```python
from build123d import *

# Parameters (mm, degrees)
SKETCH_1_R          = 2
EXTRUDE_1_DEPTH     = 8
EXTRUDE_2_DEPTH     = 39
EXTRUDE_3_DEPTH     = 35
SKETCH_4_R          = 4.5
CUT_EXTRUDE_1_DEPTH = 55
FILLET_1_R          = 1
CHAMFER_1_SIZE      = 0.2


with BuildPart() as part:
    # 草图1 → 凸台-拉伸1 (new body)
    with BuildSketch(Plane(origin=(0, 0, 0), x_dir=(0, 0, -1), z_dir=(1, 0, 0))):
        with BuildLine():
            Line((0, 4.5), (4.5, 4.5))
            Line((4.5, 4.5), (4.5, -4.5))
            Line((4.5, -4.5), (-1.5, -4.5))
            ThreePointArc((-1.5, -4.5), (-3.621320344, -3.621320344), (-4.5, -1.5))
            Line((-4.5, -1.5), (-4.5, 1.5))
            ThreePointArc((-4.5, 1.5), (-3.621320344, 3.621320344), (-1.5, 4.5))
            Line((-1.5, 4.5), (0, 4.5))
        make_face()
        Circle(SKETCH_1_R, mode=Mode.SUBTRACT)
    extrude(amount=EXTRUDE_1_DEPTH)

    # 草图2 → 凸台-拉伸2 (add)
    with BuildSketch(Plane(origin=(0, 0, -4.5), x_dir=(-1, 0, 0), z_dir=(0, 0, -1))):
        Polygon((-4, 10), (3.5, 10), (3.5, -10), (-11.5, -10), (-11.5, 10), align=None)
    extrude(amount=EXTRUDE_2_DEPTH)

    # 草图3 → 凸台-拉伸3 (add)
    with BuildSketch(Plane(origin=(0, 0, -43.5), x_dir=(-1, 0, 0), z_dir=(0, 0, -1))):
        with BuildLine():
            Line((2.5, 6.224949799), (2.5, -6.224949799))
            ThreePointArc((2.5, -6.224949799), (-4, -9), (-10.5, -6.224949799))
            Line((-10.5, -6.224949799), (-10.5, 6.224949799))
            ThreePointArc((-10.5, 6.224949799), (-4, 9), (2.5, 6.224949799))
        make_face()
    extrude(amount=EXTRUDE_3_DEPTH)

    # 草图4 → 切除-拉伸1 (cut)
    with BuildSketch(Plane(origin=(0, 0, -78.5), x_dir=(-1, 0, 0), z_dir=(0, 0, -1))):
        with Locations(Location((-4, 0, 0), (0, 0, 90))):
            Circle(SKETCH_4_R)
    extrude(amount=-CUT_EXTRUDE_1_DEPTH, mode=Mode.SUBTRACT)

    # 圆角1
    fillet_1_edges = [part.edges().sort_by_distance(p)[0] for p in [
        (4, -10, -4.5),
        (4, 10, -4.5),
        (4, 10, -43.5),
        (4, -10, -43.5),
    ]]
    fillet(fillet_1_edges, radius=FILLET_1_R - 0.0001)  # a hair under: the kernel refuses the full size

    # 倒角1
    chamfer_1_edges = [part.edges().sort_by_distance(p)[0] for p in [
        (-3.5, -10, -24),
        (11.5, -10, -24),
        (-3.5, 0, -4.5),
        (-3.5, 10, -24),
        (-3.5, 0, -43.5),
        (-3.5, 9.707136071, -4.792863929),
        (-3.5, 9.707136071, -43.207136071),
        (-3.5, -9.707136071, -43.207136071),
        (-3.5, -9.707136071, -4.792863929),
        (11.5, 0, -4.5),
        (11.5, 0, -43.5),
        (11.5, 10, -24),
        (11.5, 9.707136071, -4.792863929),
        (11.5, 9.707136071, -43.207136071),
        (11.5, -9.707136071, -43.207136071),
        (11.5, -9.707136071, -4.792863929),
    ]]
    chamfer(chamfer_1_edges, length=CHAMFER_1_SIZE)


solid = part.part
```
Verification items for the finished model (mm, model axes). A direction names the side the tool comes from. Coordinates: 2 decimals unless noted, no trailing zeros. Loops run counter-clockwise (first coordinate to the right, second up) from the corner with the lowest first, then second, coordinate; pieces in that order, holes last. Notation, with made-up numbers: (58, 2) - (66, 2) arc R13 ccw to (66, 6) - close; hole circle Ø7 at (34, -7). An arc over 180 degrees is marked (long way). Answer as a JSON object with one key per item and string values.
(1) Mould release check, pull along X, two halves, no side actions. Record for faces 4 (the cylindrical face through (4, 9, -61)), 5 (the flat face through (4, 0, -23.5)), 6 (the flat face through (9, 0, -4.5)): pulls with the +X half, pulls with the -X half, needs draft (parallel to the pull), parting line crosses it, or undercut.
Response:
{"face 4": "parting line crosses it", "face 5": "undercut", "face 6": "needs draft"}
(2) Cross-section at B-B, the plane z = 0. Record the boundary of the cut face in (x, y).
Response:
{"outline": "(0, -4.5) - (8, -4.5) - (8, -2) - (0, -2) - close; (0, 2) - (8, 2) - (8, 4.5) - (0, 4.5) - close"}
(3) Cross-section at A-A, the plane y = 0. Record the boundary of the cut face in (x, z).
Response:
{"outline": "(-3.5, -43.3) - (-3.3, -43.5) - (-2.5, -43.5) - (-2.5, -78.5) - (-0.5, -78.5) - (-0.5, -23.5) - (8.5, -23.5) - (8.5, -78.5) - (10.5, -78.5) - (10.5, -43.5) - (11.3, -43.5) - (11.5, -43.3) - (11.5, -4.7) - (11.3, -4.5) - (8, -4.5) - (8, -2) - (0, -2) - (0, -4.5) - (-3.3, -4.5) - (-3.5, -4.7) - close; (0, 2) - (8, 2) - (8, 4.5) - (0, 4.5) - close"}
(4) Scan lines: line 1 along Y through (x, z) = (2.5, 0); line 2 along X through (y, z) = (0, -35); line 3 along X through (y, z) = (-5.5, -44). Record each from-to range of solid material in increasing order.
Response:
{"line 1": "y = -4.5 to -2, 2 to 4.5", "line 2": "x = -3.5 to -0.5, 8.5 to 11.5", "line 3": "x = -2.5 to 10.5"}
(5) Access from +Z, -Z, +X, -X, +Y, -Y to the whole of each face (thin tool, end or side, straight path). Record for faces 1 (the cylindrical face through (4, -9, -61)), 2 (the flat face through (4, -4.5, -2)), 3 (the flat face through (10.5, 0, -61)).
Response:
{"face 1": "-Z, -Y", "face 2": "+Z, +X, -X, -Y", "face 3": "-Z, +X, +Y, -Y"}
(6) Go/stop test with flat-tipped pins: pin 1 Ø4.5 at (y, z) = (0, 0) entering from +X; pin 2 Ø1.5 at (y, z) = (-2, -51.5) entering from -X; pin 3 Ø5 at (x, y) = (-0.5, 4.5) entering from +Z. Record where each tip stops, or that it passes through.
Response:
{"pin 1": "stops at x = 8", "pin 2": "stops at x = -2.5", "pin 3": "stops at z = 4.45"}
(7) Cross-section at C-C, the plane z = -41.5. Record the boundary of the cut face in (x, y).
Response:
{"outline": "(-3.5, -9.8) - (-3.3, -10) - (11.3, -10) - (11.5, -9.8) - (11.5, 9.8) - (11.3, 10) - (-3.3, 10) - (-3.5, 9.8) - close; hole circle Ø9 at (4, 0)"}
